Here's the drawing with two shaded views (mm, measured from the low corner). I have some questions. Round coordinates to 2 decimals unless told otherwise and drop trailing zeros. Loops run counter-clockwise (first coordinate to the right, second up) from the corner with the lowest first, then second, coordinate; pieces in that order, holes last.
(1) Thinking about a two-plate mould opening in Z: for the marked faces 1 and 2, which applies, released by +Z, released by -Z, zero draft, split by the parting line, or undercut?
(2) I want a section at B-B on z = 4. Write out the boundary of the cut face in (x, y).
(3) I want a section at D-D on y = 15. Write out the boundary of the cut face in (x, z), plus the area to 3 significant figures.
(4) If I drill on line 1 along Y through (x, z) = (245, 7.75); line 2 along X through (y, z) = (353, 3.75); line 3 along X through (y, z) = (173, 4.25), over which ranges is the centre line in solid material (lowest first)?
(5) I want a section at A-A on y = 282. Write out the boundary of the cut face in (x, z).
(6) I want a section at C-C on x = 15. Write out the boundary of the cut face in (y, z).
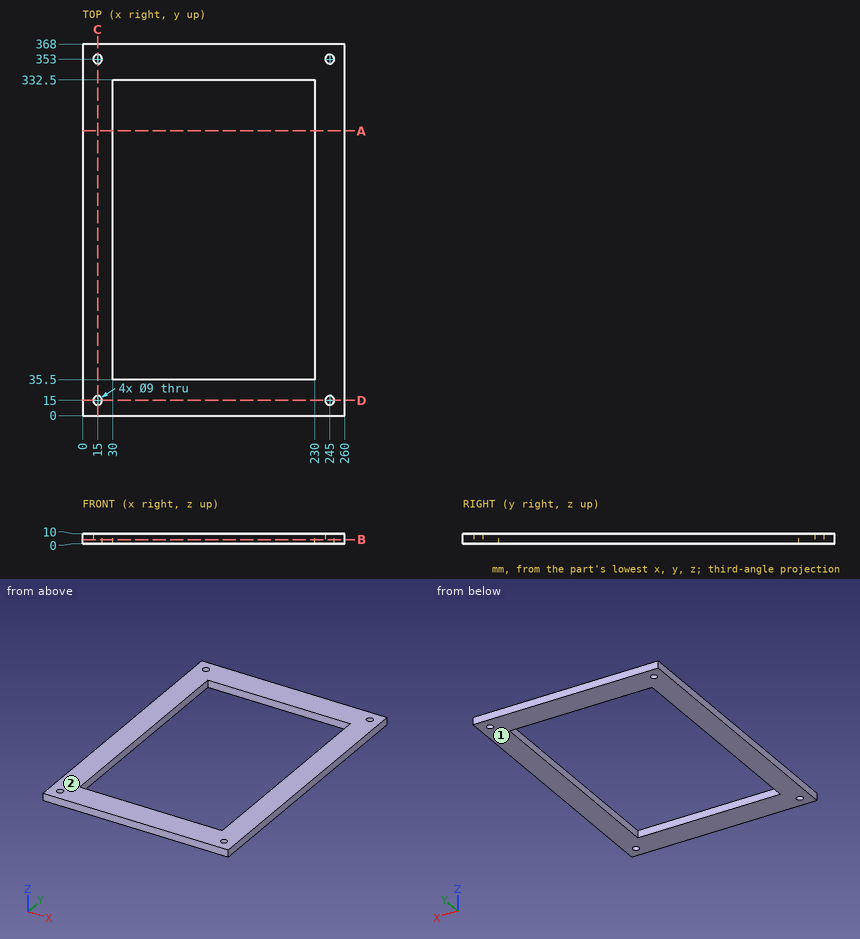
Filled sheet:
1. face 1: released by -Z
1. face 2: released by +Z
2. outline: (0, 0) - (260, 0) - (260, 368) - (0, 368) - close; hole circle Ø9 at (15, 15); hole circle Ø9 at (15, 353); hole (30, 35.5) - (230, 35.5) - (230, 332.5) - (30, 332.5) - close; hole circle Ø9 at (245, 15); hole circle Ø9 at (245, 353)
3. outline: (0, 0) - (10.5, 0) - (10.5, 10) - (0, 10) - close; (19.5, 0) - (240.5, 0) - (240.5, 10) - (19.5, 10) - close; (249.5, 0) - (260, 0) - (260, 10) - (249.5, 10) - close
3. area: 2,420 mm2
4. line 1: y = 0 to 10.5, 19.5 to 348.5, 357.5 to 368
4. line 2: x = 0 to 10.5, 19.5 to 240.5, 249.5 to 260
4. line 3: x = 0 to 30, 230 to 260
5. outline: (0, 0) - (30, 0) - (30, 10) - (0, 10) - close; (230, 0) - (260, 0) - (260, 10) - (230, 10) - close
6. outline: (0, 0) - (10.5, 0) - (10.5, 10) - (0, 10) - close; (19.5, 0) - (348.5, 0) - (348.5, 10) - (19.5, 10) - close; (357.5, 0) - (368, 0) - (368, 10) - (357.5, 10) - close
